Geometry: final body of the model. Coordinates: model frame, mm. Face numbers are marked on the shaded views. Give positions to 0.01 mm unless a question says otherwise; leave off trailing zeros. Write each loop counter-clockwise with the first axis right and the second up, starting at its lowest first coordinate (ties: lowest second). Pieces come first, ordered by that corner, then holes.
Q1. Cut plane C-C on z = 5.75. Return the cut outline in (x, y).
Q2. Pin query (flat end, axial travel): pin 1 (12 mm diameter, centred on x = 50, y = 42, fed in from +Z). Return the tip coordinate at first contact, or that it passes through.
Q3. Cut plane D-D on x = 6.5. Return the cut outline in (y, z), plus the area to 3 significant figures.
Q4. Cut plane A-A on y = -29. Return the cut outline in (x, z).
Q5. Line query: L1, parallel to Y at x = -29, z = 8.75; L2, parallel to X at y = 54, z = 5; L3, parallel to Y at x = -70, z = 4.5. Output: solid intervals per line, ascending.
Q6. Draft query along X for the marked faces 1 and 2. Return one class per face: pulls with the +X half, pulls with the -X half, needs draft (parallel to the pull), parting line crosses it, or undercut.
Q7. Cut plane B-B on x = -34. Return the cut outline in (y, z).
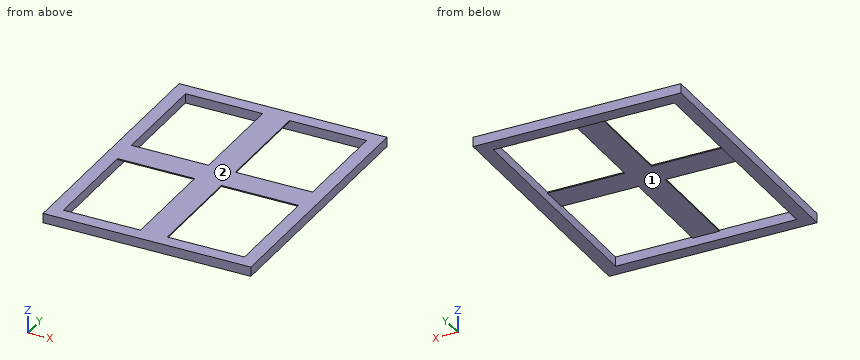
```python
from build123d import *

# Parameters (mm, degrees)
F0_W      = 196.85
F0_H      = 247.65
F0_W_2    = 171.45
F0_H_2    = 222.25
F1_DEPTH  = 9
F2_DEPTH  = 8
F3_W      = 73.025
F3_H      = 98.425
F4_DEPTH  = 9
F5_W      = 73.025
F5_H      = 98.425
F6_DEPTH  = 10
F7_W      = 73.025
F7_H      = 98.425
F8_DEPTH  = 10
F9_W      = 73.025
F9_H      = 98.425
F10_DEPTH = 10


with BuildPart() as f1:
    # F0 (on Top) → F1 (new body)
    with BuildSketch(Plane.XY):
        with Locations((-0.0278223306, 21.0249534539)):
            Rectangle(F0_W, F0_H)
        with Locations((-0.0278223306, 21.0249534539)):
            Rectangle(F0_W_2, F0_H_2, mode=Mode.SUBTRACT)
        with Locations((-0.0278223306, 21.0249534539)):
            Rectangle(F0_W_2, F0_H_2)
    extrude(amount=F1_DEPTH)

    # F0 (on Top) → F2 (cut)
    with BuildSketch(Plane.XY):
        with Locations((-0.0278223306, 21.0249534539)):
            Rectangle(F0_W_2, F0_H_2)
    extrude(amount=F2_DEPTH, mode=Mode.SUBTRACT)

    # F3 (on face) → F4 (cut)
    with BuildSketch(Plane.XY):
        with Locations((-49.2403223306, 82.9374534539)):
            Rectangle(F3_W, F3_H)
    extrude(amount=F4_DEPTH, mode=Mode.SUBTRACT)

    # F5 (on face) → F6 (cut)
    with BuildSketch(Plane(origin=(0, 0, 8), x_dir=(1, 0, 0), z_dir=(0, 0, -1))):
        with Locations((-49.2403223306, 40.8875465461)):
            Rectangle(F5_W, F5_H)
    extrude(amount=-F6_DEPTH, mode=Mode.SUBTRACT)

    # F7 (on face) → F8 (cut)
    with BuildSketch(Plane(origin=(0, 0, 8), x_dir=(1, 0, 0), z_dir=(0, 0, -1))):
        with Locations((49.1846776694, -82.9374534539)):
            Rectangle(F7_W, F7_H)
    extrude(amount=-F8_DEPTH, mode=Mode.SUBTRACT)

    # F9 (on face) → F10 (cut)
    with BuildSketch(Plane(origin=(0, 0, 8), x_dir=(1, 0, 0), z_dir=(0, 0, -1))):
        with Locations((49.1846776694, 40.8875465461)):
            Rectangle(F9_W, F9_H)
    extrude(amount=-F10_DEPTH, mode=Mode.SUBTRACT)


solid = f1.part
```
Data:
1. outline: (-98.45, -102.8) - (98.4, -102.8) - (98.4, 144.85) - (-98.45, 144.85) - close; hole (-85.75, -90.1) - (85.7, -90.1) - (85.7, 132.15) - (-85.75, 132.15) - close
2. pin 1: passes through
3. outline: (-102.8, 0) - (-90.1, 0) - (-90.1, 8) - (132.15, 8) - (132.15, 0) - (144.85, 0) - (144.85, 9) - (-102.8, 9) - close
3. area: 451 mm2
4. outline: (-98.45, 0) - (-85.75, 0) - (-85.75, 9) - (-98.45, 9) - close; (-12.73, 8) - (12.67, 8) - (12.67, 9) - (-12.73, 9) - close; (85.7, 0) - (98.4, 0) - (98.4, 9) - (85.7, 9) - close
5. L1: y = -102.8 to -90.1, 8.32 to 33.72, 132.15 to 144.85
5. L2: x = -98.45 to -85.75, 85.7 to 98.4
5. L3: y = -102.8 to -90.1, 132.15 to 144.85
6. face 1: undercut
6. face 2: needs draft
7. outline: (-102.8, 0) - (-90.1, 0) - (-90.1, 9) - (-102.8, 9) - close; (8.32, 8) - (33.72, 8) - (33.72, 9) - (8.32, 9) - close; (132.15, 0) - (144.85, 0) - (144.85, 9) - (132.15, 9) - close
